Here's how the part is built. I have some questions about the finished solid (model axes, mm). A direction names the side the tool comes from. Round coordinates to 2 decimals unless told otherwise and drop trailing zeros. Write each loop counter-clockwise with the first axis right and the second up, starting at its lowest first coordinate (ties: lowest second). Pieces come first, ordered by that corner, then holes. Notation, with made-up numbers: (-8.5, 57) -> (41.5, 57) arc R7 cw to (41.5, 67) -> close; hole circle Ø10 at (-30, 6). An arc over 180 degrees is marked (long way). Answer as CSV lines item,"result".
```python
from build123d import *

# Parameters (mm, degrees)
F0_R     = 2.033541
F1_DEPTH = 2.54


with BuildPart() as f1:
    # F0 (on Right) → F1 (new body)
    with BuildSketch(Plane.YZ):
        Polygon((11.83471, 6.069755), (0, 24.1271), (-11.83471, 6.069755), (-3.018506, -7.88928), (-11.83471, -26.197118), (0, -37.708839), (11.83471, -26.197118), (3.018506, -7.88928), align=None)
        with Locations((0, 19.871799)):
            Circle(F0_R, mode=Mode.SUBTRACT)
    extrude(amount=F1_DEPTH)


solid = f1.part
```
1. For pin 1 Ø1.5 at (x, z) = (1, 14.5) entering from +Y, with a flat end and sliding along its axis, tell me the tip position at first contact or that it passes through.
Numbers:
pin 1,"stops at y = 6.8"
2. Suppose I cut it at C-C on y = 4. Please give me the cut outline in (x, z), and give its area (3 significant figures).
Numbers:
outline,"(0, -33.82) -> (2.54, -33.82) -> (2.54, -9.93) -> (0, -9.93) -> close; (0, -6.34) -> (2.54, -6.34) -> (2.54, 18.02) -> (0, 18.02) -> close"
area,"123 mm^2"
3. Suppose I cut it at A-A on y = 7.5. Please give me the cut outline in (x, z).
Numbers:
outline,"(0, -30.41) -> (2.54, -30.41) -> (2.54, -17.2) -> (0, -17.2) -> close; (0, -0.79) -> (2.54, -0.79) -> (2.54, 12.68) -> (0, 12.68) -> close"
4. Suppose I cut it at D-D on z = -17.5. Please give me the cut outline in (x, y).
Numbers:
outline,"(0, -7.65) -> (2.54, -7.65) -> (2.54, 7.65) -> (0, 7.65) -> close"
5. If we mould it in two halves opening along Z, with no side actions, what happens to faces 4 (the face through (1.252, 5.835, -32.034)), 5 (the face through (1.252, -7.365, -16.915)), 6 (the face through (0, 0, -6))? For each: released by +Z, released by -Z, zero draft, split by the parting line, or undercut.
Numbers:
face 4,"released by -Z"
face 5,"undercut"
face 6,"zero draft"
6. If I drill on line 1 (Z direction, x = 1.1, y = -0.5); line 2 (Z direction, x = 1, y = 4.25); line 3 (Y direction, x = 0.55, z = -5), over which ranges is the centre line in solid material (lowest first)?
Numbers:
line 1,"z = -37.22 to 17.9, 21.84 to 23.36"
line 2,"z = -33.57 to -10.45, -5.94 to 17.64"
line 3,"y = -4.84 to 4.84"
7. Suppose I cut it at B-B on x = 0.7. Please give me the cut outline in (y, z), and give its area (3 significant figures).
Numbers:
outline,"(-11.83, -26.2) -> (0, -37.71) -> (11.83, -26.2) -> (3.02, -7.89) -> (11.83, 6.07) -> (0, 24.13) -> (-11.83, 6.07) -> (-3.02, -7.89) -> close; hole circle Ø4.07 at (0, 19.87)"
area,"816 mm^2"
8. On a 3-axis mill with a long thin cutter (end or side, diameter ignored), from which of +Z, -Z, +X, -X, +Y, -Y can I reach the whole of each face in a straight line? I mean faces 1 (the face through (1.252, -5.835, 15.225)), 2 (the face through (1.252, 7.365, -1.007)), 3 (the face through (1.25, -7.49, -0.81)). Say none if no direction works.
Numbers:
face 1,"+Z, +X, -X, -Y"
face 2,"+X, -X, +Y"
face 3,"+X, -X, -Y"
